from build123d import *

# Parameters (mm, degrees)
EXTRUDE_DEPTH     = 10
EXTRUDE002_DEPTH  = 10
CYLINDER016_R     = 1.6
CYLINDER016_DEPTH = 10
CYLINDER015_R     = 1.6
CYLINDER015_DEPTH = 10
CYLINDER014_R     = 1.6
CYLINDER014_DEPTH = 10
CYLINDER013_R     = 1.6
CYLINDER013_DEPTH = 10
BOX_W             = 32.2
BOX_H             = 32.2
BOX_DEPTH         = 2


with BuildPart() as extrude_body:
    # Sketch → Extrude (new body)
    with BuildSketch(Plane.XZ):
        with BuildLine():
            Line((7.9, 3.6), (6.9, 3.6))
            ThreePointArc((9.9, 6.6), (7.77868, 5.72132), (6.9, 3.6))
            Line((9.9, 6.6), (9.9, 0))
            Line((9.9, 0), (6.9, 0))
            Line((6.9, 2), (6.9, 0))
            Line((7.9, 2), (6.9, 2))
            Line((7.9, 3.6), (7.9, 2))
        make_face()
    extrude(amount=EXTRUDE_DEPTH)


with BuildPart() as part_mirroring:
    # Part__Mirroring: instance of Extrude body
    add(extrude_body.part.mirror(Plane(origin=(0, 0, 0), x_dir=(0, -1, 0), z_dir=(1, 0, 0))))


with BuildPart() as h_bridge_mount:
    # Sketch002 → Extrude002 (new body)
    with BuildSketch(Plane.XZ):
        with BuildLine():
            Line((7.9, 3.6), (6.9, 3.6))
            ThreePointArc((9.9, 6.6), (7.77868, 5.72132), (6.9, 3.6))
            Line((9.9, 6.6), (9.9, 0))
            Line((9.9, 0), (6.9, 0))
            Line((6.9, 2), (6.9, 0))
            Line((7.9, 2), (6.9, 2))
            Line((7.9, 3.6), (7.9, 2))
        make_face()
    extrude(amount=EXTRUDE002_DEPTH)

    # Fusion: union Part__Mirroring
    add(part_mirroring.part)


with BuildPart() as h_bridge_mount_1:
    # Fusion placement: moved
    add(h_bridge_mount.part.moved(Location((13, 18, 2))))


with BuildPart() as mount_point003:
    # Cylinder016 → Cylinder016 (new body)
    with BuildSketch(Plane(origin=(26, 0, 0), x_dir=(1, 0, 0), z_dir=(0, 0, 1))):
        Circle(CYLINDER016_R)
    extrude(amount=CYLINDER016_DEPTH)


with BuildPart() as mount_point002:
    # Cylinder015 → Cylinder015 (new body)
    with BuildSketch(Plane(origin=(26, 26, 0), x_dir=(1, 0, 0), z_dir=(0, 0, 1))):
        Circle(CYLINDER015_R)
    extrude(amount=CYLINDER015_DEPTH)


with BuildPart() as mount_point001:
    # Cylinder014 → Cylinder014 (new body)
    with BuildSketch(Plane(origin=(0, 26, 0), x_dir=(1, 0, 0), z_dir=(0, 0, 1))):
        Circle(CYLINDER014_R)
    extrude(amount=CYLINDER014_DEPTH)


with BuildPart() as mount_point000:
    # Cylinder013 → Cylinder013 (new body)
    with BuildSketch(Plane.XY):
        Circle(CYLINDER013_R)
    extrude(amount=CYLINDER013_DEPTH)


with BuildPart() as fusion001:
    # Box → Box (new body)
    with BuildSketch(Plane(origin=(-3.1, -3.1, 0), x_dir=(1, 0, 0), z_dir=(0, 0, 1))):
        with Locations((16.1, 16.1)):
            Rectangle(BOX_W, BOX_H)
    extrude(amount=BOX_DEPTH)

    # Cut: cut Mount Point000
    add(mount_point000.part, mode=Mode.SUBTRACT)

    # Cut001: cut Mount Point001
    add(mount_point001.part, mode=Mode.SUBTRACT)

    # Cut002: cut Mount Point002
    add(mount_point002.part, mode=Mode.SUBTRACT)

    # Cut003: cut Mount Point003
    add(mount_point003.part, mode=Mode.SUBTRACT)

    # Fusion001: union H Bridge Mount
    add(h_bridge_mount_1.part)


solid = fusion001.part
Source: CAD feature listing. Evaluate the final solid. Frame: model axes, mm. A direction names the side the tool comes from. Coordinates: 2 decimals unless noted, no trailing zeros. Loops run counter-clockwise (first coordinate to the right, second up) from the corner with the lowest first, then second, coordinate; pieces in that order, holes last. Notation, with made-up numbers: (46.25, -31.75) - (56.25, -31.75) arc R25 ccw to (56.25, 0.25) - close; hole circle Ø3 at (-21.75, 89). An arc over 180 degrees is marked (long way). Return JSON: item names as keys, results as strings.
Q1. Contact query for flat-ended pins moving along their axis: P1, Ø3, axis at x = 0, y = 0, coming from the +Z side; P2, Ø1.5, axis at y = 9, z = 7, coming from the +X side; P3, Ø5, axis at x = 26, y = 26, coming from the +Z side; P4, Ø1.5, axis at x = 5.5, z = 4.5, coming from the -Y side. Output: stop coordinate, or through.
Results:
{"P1": "through", "P2": "x = 22.9", "P3": "z = 2", "P4": "y = 8"}
Q2. Material intervals for line 1 along Y through (x, z) = (0, 1.65); line 2 along Z through (x, y) = (13, 20.5), sorted ascending.
Results:
{"line 1": "-3.1 to -1.6, 1.6 to 24.4, 27.6 to 29.1", "line 2": "0 to 2"}
Q3. Section D-D, the plane z = 0.75. Return loops of the section in (x, y).
Results:
{"outline": "(-3.1, -3.1) - (29.1, -3.1) - (29.1, 29.1) - (-3.1, 29.1) - close; hole circle Ø3.2 at (0, 0); hole circle Ø3.2 at (0, 26); hole circle Ø3.2 at (26, 0); hole circle Ø3.2 at (26, 26)"}
Q4. Access query for faces 4 (the flat face through (4, 18, 5)), 5 (the cylindrical face through (5.2, 13.07, 7.74)), 6 (the flat face through (22.9, 13, 5)), 7 (the flat face through (22, 8, 5)), 8 (the flat face through (5.6, 13.1, 4)). Directions: +Z, -Z, +X, -X, +Y, -Y. A direction counts if a zero-diameter tool reaches every point of the face in a straight line with its end or side. Return the directions, or none.
Results:
{"face 4": "+Z, +X, -X, +Y", "face 5": "+Z, +Y, -Y", "face 6": "+Z, +X, +Y, -Y", "face 7": "+Z, +X, -X, -Y", "face 8": "+Y, -Y"}
Q5. Section B-B, the plane y = 26. Return loops of the section in (x, z), plus the area to 3 significant figures.
Results:
{"outline": "(-3.1, 0) - (-1.6, 0) - (-1.6, 2) - (-3.1, 2) - close; (1.6, 0) - (24.4, 0) - (24.4, 2) - (1.6, 2) - close; (27.6, 0) - (29.1, 0) - (29.1, 2) - (27.6, 2) - close", "area": "51.6 mm2"}
Q6. Mould query, pull axis Z, two halves, no side actions, for faces 1 (the flat face through (20.4, 13.1, 4)), 2 (the flat face through (13, 29.1, 1)), 3 (the flat face through (13, 13, 0)). Classes: released by +Z, released by -Z, zero draft, split by the parting line, or undercut.
Results:
{"face 1": "undercut", "face 2": "zero draft", "face 3": "released by -Z"}
Q7. Section A-A, the plane z = 5. Return loops of the section in (x, y).
Results:
{"outline": "(3.1, 8) - (5.1, 8) - (5.1, 18) - (3.1, 18) - close; (20.9, 8) - (22.9, 8) - (22.9, 18) - (20.9, 18) - close"}
